from build123d import *

# Parameters (mm, degrees)
F0_R          = 25.4
F1_DEPTH      = 63.5
F1_DEPTH_BACK = 53.975
F3_DEPTH      = 50.8


with BuildPart() as f1:
    # F0 (on Front) → F1 (new body, two sides)
    with BuildSketch(Plane.XZ) as f1_sk:
        with BuildLine():
            ThreePointArc((-20.777584, 18.864096), (0, 12.7), (20.777584, 18.864096))
            ThreePointArc((20.777584, 18.864096), (33.490566, 32.634318), (38.1, 50.8))
            ThreePointArc((38.1, 50.8), (-18.165682, 84.290566), (-20.777584, 18.864096))
        make_face()
        with Locations((0, 50.8)):
            Circle(F0_R, mode=Mode.SUBTRACT)
        with BuildLine():
            ThreePointArc((-36.801774, -40.938994), (0, -12.7), (36.801774, -40.938994))
            Line((36.801774, -40.938994), (20.777584, 18.864096))
            ThreePointArc((20.777584, 18.864096), (0, 12.7), (-20.777584, 18.864096))
            Line((-20.777584, 18.864096), (-36.801774, -40.938994))
        make_face()
        with BuildLine():
            ThreePointArc((-36.801774, -40.938994), (-4.973048, -88.574049), (38.1, -50.8))
            ThreePointArc((38.1, -50.8), (37.774049, -45.826952), (36.801774, -40.938994))
            ThreePointArc((36.801774, -40.938994), (0, -12.7), (-36.801774, -40.938994))
        make_face()
        with Locations((0, -50.8)):
            Circle(F0_R, mode=Mode.SUBTRACT)
    extrude(amount=F1_DEPTH)
    extrude(f1_sk.sketch, amount=-F1_DEPTH_BACK)

    # F2 (on Right) → F3 (intersect, symmetric)
    with BuildSketch(Plane.YZ):
        Polygon((0, 88.9), (-63.5, 88.9), (12.7, -43.082272), (12.7, -88.9), (53.975, -88.9), (0, 4.587442), align=None)
    extrude(amount=F3_DEPTH, both=True, mode=Mode.INTERSECT)


solid = f1.part
The listing builds one solid part. Answer for the finished solid, in the listing's coordinates (mm). A direction names the side the tool comes from. Coordinates: 2 decimals unless noted, no trailing zeros. Order: outer loops, then holes, each group sorted by start corner. A loop starts at its lowest first (then second) coordinate and runs counter-clockwise, first axis right, second up.
Q1. Given P1, Ø23, axis at x = 15, z = -63.5, coming from the -Y side; P2, Ø1, axis at x = 7, z = 21.5, coming from the -Y side; P3, Ø12, axis at y = -11, z = 68, coming from the -X side, each flat-ended and moving along its own axis, determine where each tip first touches the part or whether it passes through.
Q2. A cutting plane is placed at C-C, the plane x = 0. Write down the section's boundary in (y, z) (3 decimals).
Q3. Consider line 1 (X direction, y = 25, z = -50); line 2 (Z direction, x = 0, y = 20.5); line 3 (X direction, y = -37, z = 57.5). Determine where each line is inside the solid, lowest interval first.
Q4. A cutting plane is placed at D-D, the plane y = -19. Write down the section's boundary in (x, z), and give its area (3 significant figures).
Q5. A cutting plane is placed at B-B, the plane x = 32.5. Write down the section's boundary in (y, z), and give its area (3 significant figures).
Q6. For a pull along Z with two mould halves and no side action, classify faces 5 (the face through (37.783, 21.577, -45.896)), 6 (the face through (17, 0, 27)), 7 (the face through (-3.307, -21.45, 75.984)), 8 (the face through (0.53, -25.93, 23.83)) as pulls with the +Z half, pulls with the -Z half, needs draft (parallel to the pull), parting line crosses it, or undercut.
Q7. A cutting plane is placed at A-A, the plane z = -34.5. Write down the section's boundary in (x, y), and give its area (3 significant figures).
Q8. Which of the six approach directions +Z, -Z, +X, -X, +Y, -Y give full straight-line access (tool end or side, diameter ignored) to faces 1 (the face through (9, 12.7, -76)), 2 (the face through (28.234, 3.323, -8.962)), 3 (the face through (-5.506, 24.163, -75.596)), 4 (the face through (-28.16, -0.33, -8.68))?
Answers follow:
1. P1: stops at y = 12.7
1. P2: stops at y = -24.88
1. P3: stops at x = -36.42
2. outline: (-63.5, 88.9) - (-56.168, 76.2) - (0, 76.2) - (0, 88.9) - close; (-26.838, 25.4) - (2.491, -25.4) - (17.313, -25.4) - (0, 4.587) - (0, 25.4) - close; (12.7, -88.9) - (53.975, -88.9) - (46.643, -76.2) - (12.7, -76.2) - close
3. line 1: x = -38.09 to -25.39, 25.39 to 38.09
3. line 2: z = -88.9 to -76.2
3. line 3: x = -37.51 to -24.5, 24.5 to 37.51
4. outline: (-22.66, 11.82) - (22.66, 11.82) - (20.78, 18.86) arc R38.1 ccw to (38.1, 50.8) arc R38.1 ccw (long way) to (-20.78, 18.86) - close; hole circle Ø50.8 at (0, 50.8)
4. area: 2,670 mm2
5. outline: (-52.98, 70.68) - (-30.02, 30.92) - (0, 30.92) - (0, 70.68) - close; (2.19, -24.88) - (12.7, -43.08) - (12.7, -70.68) - (43.46, -70.68) - (17.02, -24.88) - close
5. area: 2,550 mm2
6. face 5: pulls with the +Z half
6. face 6: needs draft
6. face 7: undercut
6. face 8: pulls with the -Z half
7. outline: (-35.08, 7.75) - (-19.48, 7.75) - (-19.48, 22.57) - (-35.08, 22.57) - close; (19.48, 7.75) - (35.08, 7.75) - (35.08, 22.57) - (19.48, 22.57) - close
7. area: 462 mm2
8. face 1: -Z, +X, -X, -Y
8. face 2: +X, +Y, -Y
8. face 3: +Y, -Y
8. face 4: -X, +Y, -Y
